from build123d import *

# Parameters (mm, degrees)
F1_DEPTH       = 30
F2_R           = 0.5
F4_D           = 3.5
F4_CSINK_D     = 6.8
F4_CSINK_ANGLE = 90


with BuildPart() as f1:
    # F0 (on Top) → F1 (new body)
    with BuildSketch(Plane.XY):
        Polygon((0, 30), (0, 0), (5, 0), (5, 22), (2, 22), (2, 30), align=None)
    extrude(amount=F1_DEPTH)

    # F2
    f2_edges = [f1.edges().sort_by_distance(p)[0] for p in [
        (2, 30, 15),
        (2, 26, 0),
        (3.5, 22, 0),
        (5, 11, 0),
        (5, 0, 15),
        (2, 26, 30),
        (5, 22, 15),
        (5, 11, 30),
        (3.5, 22, 30),
        (1, 30, 30),
        (2.5, 0, 30),
        (2.5, 0, 0),
        (0, 15, 0),
        (0, 15, 30),
        (0, 30, 15),
        (0, 0, 15),
    ]]
    fillet(f2_edges, radius=F2_R)

    # F4 (through all)
    with Locations(Plane(origin=(0, 0, 0), x_dir=(0, -1, 0), z_dir=(-1, 0, 0))):
        with Locations((-11.5, 15)):
            CounterSinkHole(F4_D / 2, F4_CSINK_D / 2, counter_sink_angle=F4_CSINK_ANGLE)


solid = f1.part
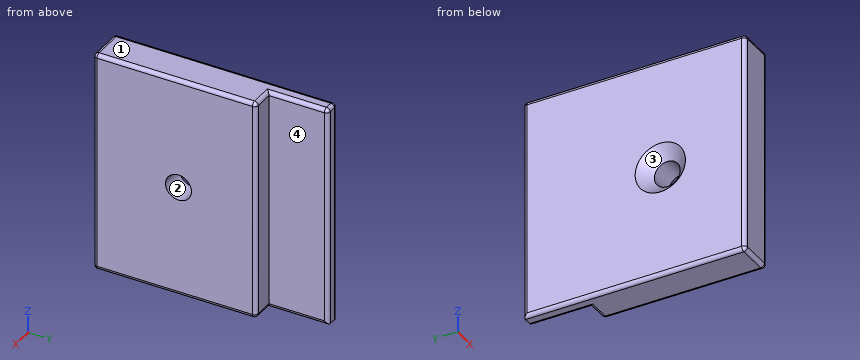
Input: part model. Units: mm. Frame: model coordinates. Face numbers are marked on the shaded views. Round coordinates to 2 decimals unless told otherwise and drop trailing zeros. Order: outer loops, then holes, each group sorted by start corner. A loop starts at its lowest first (then second) coordinate and runs counter-clockwise, first axis right, second up. Notation, with made-up numbers: (73, -9) - (93, -9) arc R7 ccw to (93, -5) - close; hole circle Ø11 at (25, 25). An arc over 180 degrees is marked (long way). Use a Markdown table: item, result.
1. Material intervals for probe 1 along Z at (x, y) = (3.05, 11.5); probe 2 along Y at (x, z) = (3.6, 15); probe 3 along Y at (x, z) = (2.5, 17.25), sorted ascending.
Evaluation:
| item | result |
|---|---|
| probe 1 | 0 to 13.25, 16.75 to 30 |
| probe 2 | 0 to 9.75, 13.25 to 22 |
| probe 3 | 0 to 22 |
2. Section B-B on z = 15. Return the cut outline in (x, y), then the cut area to 3 significant figures.
Evaluation:
| item | result |
|---|---|
| outline | (0, 0.5) arc R0.5 ccw to (0.5, 0) - (4.5, 0) arc R0.5 ccw to (5, 0.5) - (5, 9.75) - (1.65, 9.75) - (0, 8.1) - close; (0, 14.9) - (1.65, 13.25) - (5, 13.25) - (5, 21.5) arc R0.5 ccw to (4.5, 22) - (2, 22) - (2, 29.5) arc R0.5 ccw to (1.5, 30) - (0.5, 30) arc R0.5 ccw to (0, 29.5) - close |
| area | 106 mm^2 |
3. Section A-A on y = 11.5. Return the cut outline in (x, z).
Evaluation:
| item | result |
|---|---|
| outline | (0, 0.5) arc R0.5 ccw to (0.5, 0) - (4.5, 0) arc R0.5 ccw to (5, 0.5) - (5, 13.25) - (1.65, 13.25) - (0, 11.6) - close; (0, 18.4) - (1.65, 16.75) - (5, 16.75) - (5, 29.5) arc R0.5 ccw to (4.5, 30) - (0.5, 30) arc R0.5 ccw to (0, 29.5) - close |
4. Mould query, pull axis Z, two halves, no side actions, for the marked faces 1, 2, 3 and 4. Classes: +Z half, -Z half, draft (parallel to the pull), parting line (faces both ways), or undercut.
Evaluation:
| item | result |
|---|---|
| face 1 | +Z half |
| face 2 | undercut |
| face 3 | undercut |
| face 4 | draft |
5. Section D-D on y = 22.5. Return the cut outline in (x, z).
Evaluation:
| item | result |
|---|---|
| outline | (0, 0.5) arc R0.5 ccw to (0.5, 0) - (1.5, 0) arc R0.5 ccw to (2, 0.5) - (2, 29.5) arc R0.5 ccw to (1.5, 30) - (0.5, 30) arc R0.5 ccw to (0, 29.5) - close |
6. First-contact query: pin 1 (6 mm diameter, centred on y = 27, z = 18, fed in from +X); pin 2 (0.8 mm diameter, centred on x = 3, z = 21, fed in from +Y). Flat tips, straight axial feed; report the tip coordinate or a pass-through.
Evaluation:
| item | result |
|---|---|
| pin 1 | x = 2 |
| pin 2 | y = 22 |
7. Section C-C on x = 2.75. Return the cut outline in (y, z), then the cut area to 3 significant figures.
Evaluation:
| item | result |
|---|---|
| outline | (0, 0.5) arc R0.5 ccw to (0.5, 0) - (21.5, 0) arc R0.5 ccw to (22, 0.5) - (22, 29.5) arc R0.5 ccw to (21.5, 30) - (0.5, 30) arc R0.5 ccw to (0, 29.5) - close; hole circle Ø3.5 at (11.5, 15) |
| area | 650 mm^2 |
